Answer from the drawing. Dimensions are ordinates in mm from the lowest x, y and z of the part. A direction names the side the tool comes from. Give positions to 0.01 mm unless a question says otherwise; leave off trailing zeros. Loops run counter-clockwise (first coordinate to the right, second up) from the corner with the lowest first, then second, coordinate; pieces in that order, holes last. Notation, with made-up numbers: M -36,63 L 7,63 A9 cw 7,73 Z; hole C 71.5,-1.5 d8. An arc over 180 degrees is marked long. Use a Markdown table: item, result.
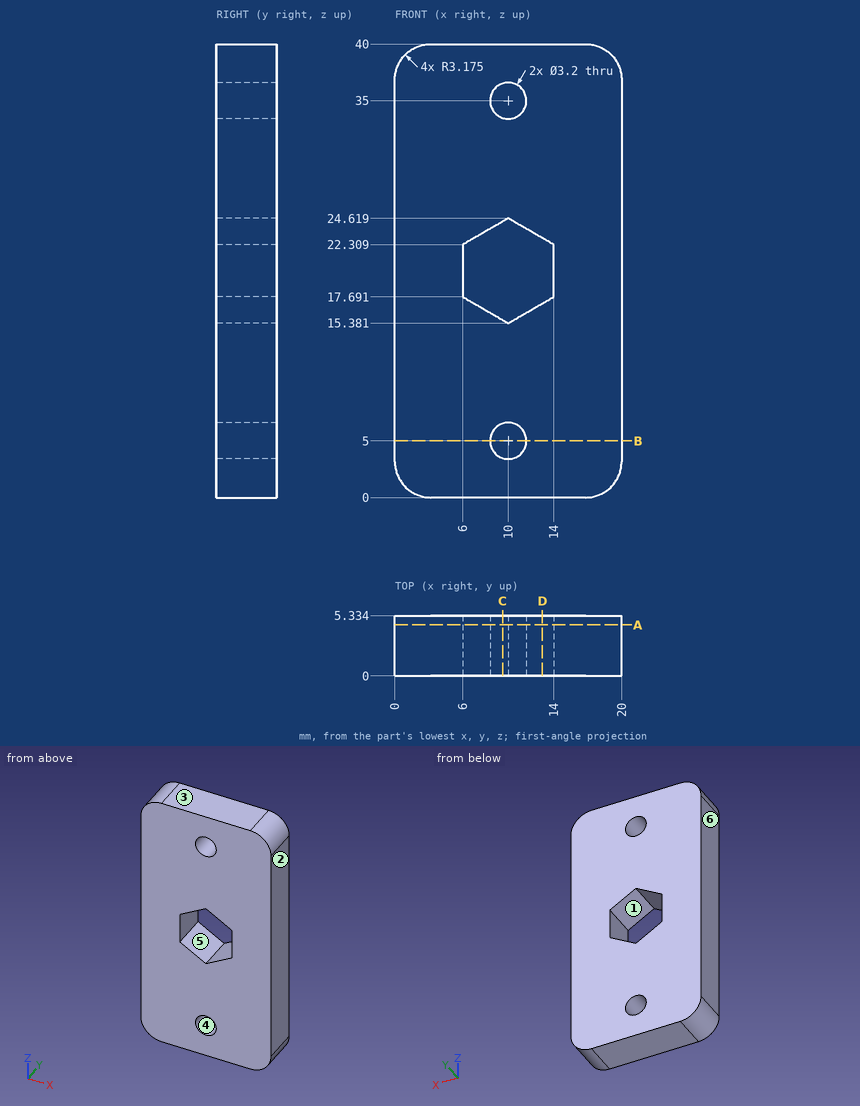
(1) A cutting plane is placed at D-D (x = 13). Write down the section's boundary in (y, z).
Entries:
| item | result |
|---|---|
| outline | M 0,0 L 5.33,0 L 5.33,17.11 L 0,17.11 Z; M 0,22.89 L 5.33,22.89 L 5.33,40 L 0,40 Z |
(2) A cutting plane is placed at C-C (x = 9.5). Write down the section's boundary in (y, z).
Entries:
| item | result |
|---|---|
| outline | M 0,0 L 5.33,0 L 5.33,3.48 L 0,3.48 Z; M 0,6.52 L 5.33,6.52 L 5.33,15.67 L 0,15.67 Z; M 0,24.33 L 5.33,24.33 L 5.33,33.48 L 0,33.48 Z; M 0,36.52 L 5.33,36.52 L 5.33,40 L 0,40 Z |
(3) Which of the six approach directions +Z, -Z, +X, -X, +Y, -Y give full straight-line access (tool end or side, diameter ignored) to the marked faces 5 and 6?
Entries:
| item | result |
|---|---|
| face 5 | +Y, -Y |
| face 6 | +Z, -Z, -X, +Y, -Y |
(4) Consider probe 1 along Z at (x, y) = (10, 1.7); probe 2 along X at (y, z) = (2.75, 20); probe 3 along X at (y, z) = (2.65, 35). Determine where each line is inside the solid, lowest interval first. Write a range as [from, to].
Entries:
| item | result |
|---|---|
| probe 1 | z = [0, 3.4], [6.6, 15.38], [24.62, 33.4], [36.6, 40] |
| probe 2 | x = [0, 6], [14, 20] |
| probe 3 | x = [0, 8.4], [11.6, 20] |
(5) A cutting plane is placed at A-A (y = 4.5). Count the separate pieces of the cut face and the enclosed holes in it, and give its area (3 significant figures).
Entries:
| item | result |
|---|---|
| separate pieces | 1 |
| enclosed holes | 3 |
| area | 720 mm² |
(6) The mould has two halves that part along X. Classify the marked faces 1, 2, 3 and 4: released by +X, released by -X, zero draft, split by the parting line, or undercut.
Entries:
| item | result |
|---|---|
| face 1 | undercut |
| face 2 | released by +X |
| face 3 | zero draft |
| face 4 | undercut |
(7) A cutting plane is placed at B-B (z = 5). Write down the section's boundary in (x, y).
Entries:
| item | result |
|---|---|
| outline | M 0,0 L 8.4,0 L 8.4,5.33 L 0,5.33 Z; M 11.6,0 L 20,0 L 20,5.33 L 11.6,5.33 Z |
